Part print with two shaded views. Sizes in mm from the minimum x, y, z corner. A direction names the side the tool comes from. Give positions to 0.01 mm unless a question says otherwise; leave off trailing zeros. Loops run counter-clockwise (first coordinate to the right, second up) from the corner with the lowest first, then second, coordinate; pieces in that order, holes last. Notation, with made-up numbers: M 20,27.25 L 59,27.25 A23 cw 59,43.25 Z; hole C -18,69 d9. An arc over 180 degrees is marked long. Answer as a JSON object with one key per item and string values. Group by question number.
1. Slice it at A-A (y = 14). Give the number of separate pieces and of enclosed holes in the cut face, then the cut area to 3 significant figures.
2. Slice it at C-C (z = 27). List the corners of the cut face in (x, y) (1 decimal), then the cut area to 3 significant figures.
3. Drill centre lines: line 1 along X through (y, z) = (12.75, 10); line 2 along Y through (x, z) = (57, 10.5); line 3 along Z through (x, y) = (12.7, 12.5). Where is each one in solid material? Low to high. Write a range as [from, to].
4. 3-axis set-ups, long thin cutter, end or side, ignore diameter. For the marked faces 1, 2 and 3: which of +Z, -Z, +X, -X, +Y, -Y reach the whole face in a straight line?
5. Mould opens along X. For the marked faces 4, 5 and 6 say: released by +X, released by -X, zero draft, split by the parting line, or undercut.
6. Drop flat-ended pins along their axis: pin 1 Ø12.5 at (x, y) = (57, 16.5) entering from +Z; pin 2 Ø4 at (y, z) = (19, 21.5) entering from +X; pin 3 Ø1 at (y, z) = (13, 33) entering from +X. Give the stop position or say it passes through.
7. Slice it at D-D (z = 7.5). List the corners of the cut face in (x, y).
8. Slice it at B-B (x = 50). List the corners of the cut face in (y, z).
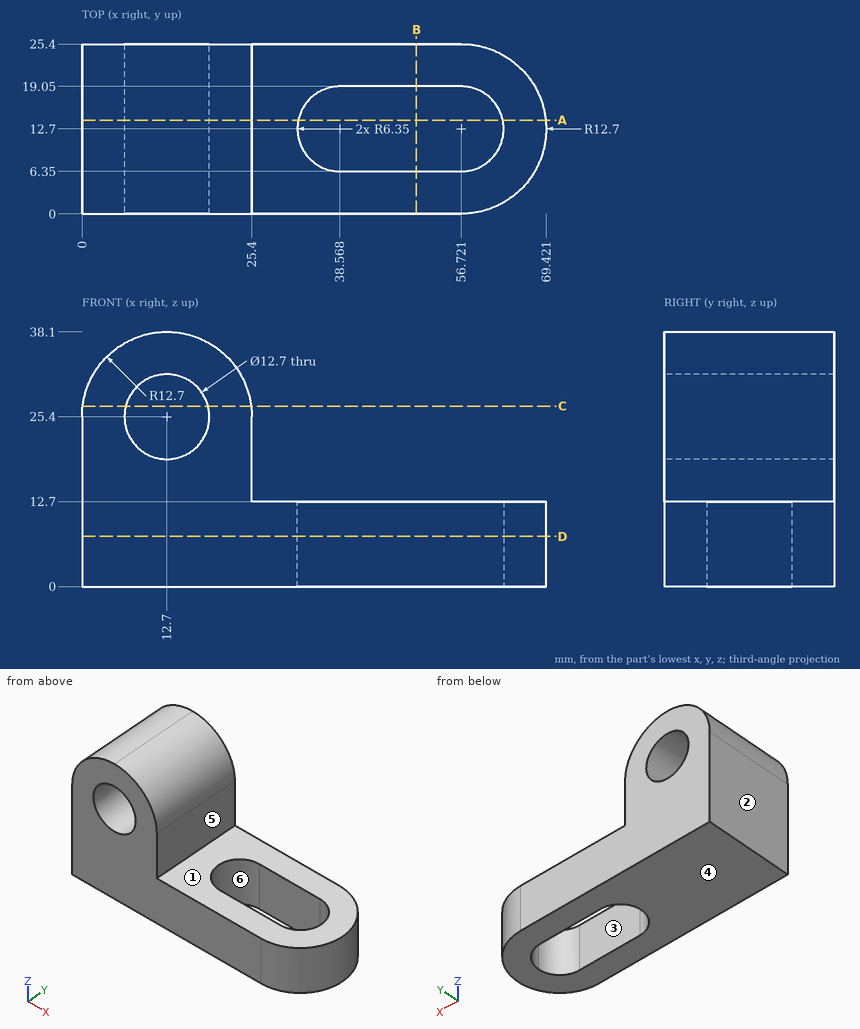
Established:
{
 "1": {"separate pieces": "2", "enclosed holes": "1", "area": "942 mm^2"},
 "2": {"outline": "M 0.1,0 L 6.6,0 L 6.6,25.4 L 0.1,25.4 Z; M 18.8,0 L 25.3,0 L 25.3,25.4 L 18.8,25.4 Z", "area": "328 mm^2"},
 "3": {"line 1": "x = [0, 32.22], [63.07, 69.42]", "line 2": "y = [0, 6.36], [19.04, 25.4]", "line 3": "z = [0, 19.05], [31.75, 38.1]"},
 "4": {"face 1": "+Z, +X, +Y, -Y", "face 2": "+Z, -Z, -X, +Y, -Y", "face 3": "+Z, -Z"},
 "5": {"face 4": "zero draft", "face 5": "released by +X", "face 6": "undercut"},
 "6": {"pin 1": "stops at z = 12.7", "pin 2": "stops at x = 25.4", "pin 3": "stops at x = 23.23"},
 "7": {"outline": "M 0,0 L 56.72,0 A12.7 ccw 56.72,25.4 L 0,25.4 Z; hole M 38.57,6.35 L 56.72,6.35 A6.35 ccw 56.72,19.05 L 38.57,19.05 A6.35 ccw Z"},
 "8": {"outline": "M 0,0 L 6.35,0 L 6.35,12.7 L 0,12.7 Z; M 19.05,0 L 25.4,0 L 25.4,12.7 L 19.05,12.7 Z"}
}
